Design review of the part built by this model. Coordinates are the model's own, in mm. A direction names the side the tool comes from. Coordinates: 2 decimals unless noted, no trailing zeros. Loops run counter-clockwise (first coordinate to the right, second up) from the corner with the lowest first, then second, coordinate; pieces in that order, holes last. Notation, with made-up numbers: (89, 40.25) -> (101, 40.25) arc R18 cw to (101, 68.25) -> close; hole circle Ø2 at (75, 57.5). An arc over 180 degrees is marked (long way). Answer as a JSON object with one key per item and string values.
```python
from build123d import *

# Parameters (mm, degrees)
F0_W = 1524
F0_H = 127
F2_W = 762
F2_H = 305.5362462927


# Not quite as in the source:
# - a fillet or chamfer that OpenCascade refuses, or shapes differently, is made with other operations: its cross-section is extruded or revolved along the edge and cut away or added


with BuildPart() as f1:
    # F0 (on Front) → F1 (revolve)
    with BuildSketch(Plane.XZ):
        with Locations((128.8676711868, 63.5)):
            Rectangle(F0_W, F0_H)
    revolve(axis=Axis((128.8676711868, 0, 0), (1, 0, 0)))

    # F2 (on Front) → F3 (revolve, cut)
    with BuildSketch(Plane.XZ):
        with Locations((132.5217391304, 241.6681231464)):
            Rectangle(F2_W, F2_H)
    revolve(axis=Axis((22.0869673282, 0, 0), (1, 0, 0)), mode=Mode.SUBTRACT)

    # F4: fillet of radius 127 on 1 edges, made by hand

    # F4_s1 → F4_t2 (revolve)
    with BuildSketch(Plane.XZ):
        with BuildLine():
            ThreePointArc((-248.4782608696, 127), (-206.9690083239, 98.8117853924), (-157.7821198271, 88.9))
            Line((-157.7821198271, 88.9), (-248.4782608696, 88.9))
            Line((-248.4782608696, 88.9), (-248.4782608696, 127))
        make_face()
    revolve(axis=Axis((-248.4782608696, 0, 0), (1, 0, 0)))

    # F5: fillet of radius 127 on 1 edges, made by hand

    # F5_s1 → F5_t2 (revolve)
    with BuildSketch(Plane.XZ):
        with BuildLine():
            ThreePointArc((422.8255980879, 88.9), (472.0124865848, 98.8117853924), (513.5217391304, 127))
            Line((513.5217391304, 127), (513.5217391304, 88.9))
            Line((513.5217391304, 88.9), (422.8255980879, 88.9))
        make_face()
    revolve(axis=Axis((513.5217391304, 0, 0), (1, 0, 0)))


solid = f1.part
```
1) For faces 1 (the cylindrical face through (136.586, -26.703, 84.795)), 2 (the flat face through (-633.132, -2, 2)), list the 3-axis set-ups (+Z, -Z, +X, -X, +Y, -Y) from which the entire face can be reached by the end or side of a thin tool; tool diameter is ignored.
Completed:
{"face 1": "none", "face 2": "+Z, -Z, -X, +Y, -Y"}
2) Add section A-A, the plane z = 0. Give the boundary of the cut face in (x, y), and give its area (3 significant figures).
Completed:
{"outline": "(-633.13, -127) -> (-248.48, -127) arc R127 cw to (-157.78, -88.9) -> (422.83, -88.9) arc R127 cw to (513.52, -127) -> (890.87, -127) -> (890.87, 127) -> (513.52, 127) arc R127 cw to (422.83, 88.9) -> (-157.78, 88.9) arc R127 cw to (-248.48, 127) -> (-633.13, 127) -> close", "area": "333,000 mm²"}
3) Clearance check with flat-ended pins moving along their axes: pin 1 Ø4 at (x, y) = (215.5, 16.5) entering from -Z; pin 2 Ø4 at (y, z) = (84.5, -98) entering from +X; pin 3 Ø10 at (x, z) = (-159.5, 30.5) entering from +Y; pin 4 Ø3 at (x, y) = (-302.5, -91.5) entering from +Z. State where each tip first meets the part, or that it passes through.
Completed:
{"pin 1": "z = -87.71", "pin 2": "through", "pin 3": "y = 85.18", "pin 4": "z = 89.6"}
4) Add section C-C, the plane x = 667. Give the boundary of the cut face in (y, z).
Completed:
{"outline": "circle Ø254 at (0, 0)"}
5) Add section D-D, the plane x = 47. Give the boundary of the cut face in (y, z).
Completed:
{"outline": "circle Ø177.8 at (0, 0)"}
6) Wall thickness on probe 1 along Y at (x, z) = (-444.5, 1.5); probe 2 along X at (y, z) = (100, -55); probe 3 along X at (y, z) = (94.5, -41.5): over which ranges is each line inside the solid? List them lowest first.
Completed:
{"probe 1": "-126.99 to 126.99", "probe 2": "-633.13 to -233.75, 498.79 to 890.87", "probe 3": "-633.13 to -216.35, 481.39 to 890.87"}
